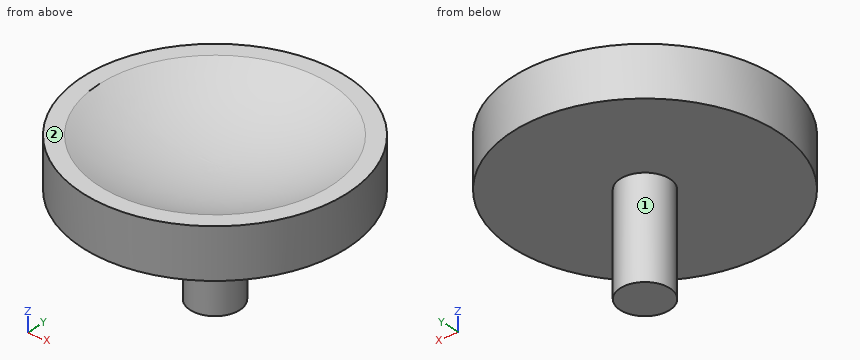
```python
from build123d import *

# Parameters (mm, degrees)
F0_R     = 10.16
F1_DEPTH = 3.81
F4_R     = 1.905
F5_DEPTH = 7.62


with BuildPart() as f1:
    # F0 (on Top) → F1 (new body)
    with BuildSketch(Plane.XY):
        Circle(F0_R)
    extrude(amount=F1_DEPTH)

    # F2 (on Front) → F3 (revolve, cut)
    with BuildSketch(Plane.XZ):
        with BuildLine():
            Line((0, 3.81), (-8.89, 3.81))
            ThreePointArc((-8.89, 3.81), (-4.559636, 2.292467), (0, 1.778))
            Line((0, 1.778), (0, 3.81))
        make_face()
    revolve(axis=Axis((0, 0, 2.794), (0, 0, -1)), mode=Mode.SUBTRACT)

    # F4 (on face) → F5 (join)
    with BuildSketch(Plane(origin=(0, 0, 0), x_dir=(1, 0, 0), z_dir=(0, 0, -1))):
        Circle(F4_R)
    extrude(amount=F5_DEPTH)


solid = f1.part
```
CAD build for the part. Positions are in the model's coordinates, mm. Face numbers are marked on the shaded views. A direction names the side the tool comes from. Round coordinates to 2 decimals unless told otherwise and drop trailing zeros. Loops run counter-clockwise (first coordinate to the right, second up) from the corner with the lowest first, then second, coordinate; pieces in that order, holes last. Notation, with made-up numbers: (32, 85) - (61, 85) arc R32 ccw to (61, 118) - close; hole circle Ø11 at (67.5, 72.5). An arc over 180 degrees is marked (long way). Return JSON: item names as keys, results as strings. Group by question number.
Q1. Flat gauge pins, fed straight in: pin 1 Ø1 at (y, z) = (7, 2) entering from -X; pin 2 Ø5 at (x, z) = (-3.5, -1) entering from -Y; pin 3 Ø2 at (x, y) = (-7.5, -2) entering from -Z. Where does each tip first touch, or does it go through?
Q2. Band-saw the part on A-A on z = -3.5. Give the cut face in (x, y) (3 decimals), plus the area to 3 significant figures.
Q3. Drill centre lines: line 1 along Z through (x, y) = (-5.5, 7); line 2 along Z through (x, y) = (2, 2.25); line 3 along Y through (x, z) = (5.75, 2). Where is each one in solid material? Low to high. Write a range as [from, to].
Q4. Tool access for the marked faces 1 and 2: list every direction of +Z, -Z, +X, -X, +Y, -Y with a clear straight run to the whole face (end or side of a thin tool).
Solutions:
{
 "1": {"pin 1": "stops at x = -7.81", "pin 2": "stops at y = -10.09", "pin 3": "stops at z = 0"},
 "2": {"outline": "circle Ø3.81 at (0, 0)", "area": "11.4 mm^2"},
 "3": {"line 1": "z = [0, 3.81]", "line 2": "z = [0, 2]", "line 3": "y = [-8.38, 8.38]"},
 "4": {"face 1": "-Z", "face 2": "+Z, +X, -X, +Y, -Y"}
}
